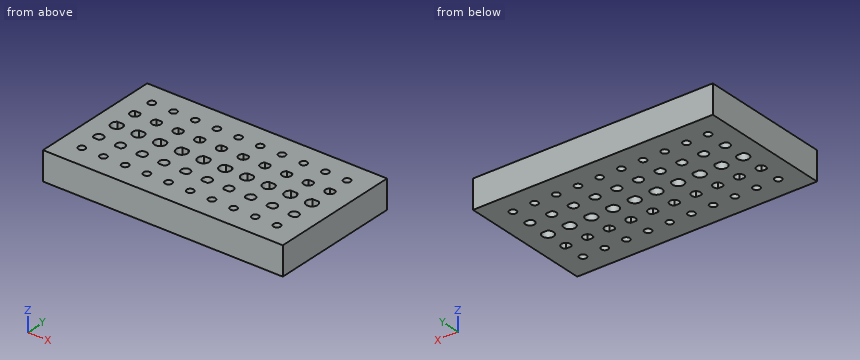
from build123d import *

# Parameters (mm, degrees)
F1_W     = 210
F1_H     = 116
F1_R     = 3.05
F2_DEPTH = 25


with BuildPart() as f2:
    # F1 (on face) → F2 (new body)
    with BuildSketch(Plane.XY):
        with Locations((105, 58)):
            Rectangle(F1_W, F1_H)
        with Locations((19, 19)):
            Circle(F1_R, mode=Mode.SUBTRACT)
        with Locations((38, 19)):
            Circle(F1_R, mode=Mode.SUBTRACT)
        with Locations((57, 19)):
            Circle(F1_R, mode=Mode.SUBTRACT)
        with Locations((76, 19)):
            Circle(F1_R, mode=Mode.SUBTRACT)
        with Locations((95, 19)):
            Circle(F1_R, mode=Mode.SUBTRACT)
        with BuildLine():
            Line((21.362954, 34.834728), (16.637046, 34.834728))
            ThreePointArc((16.637046, 34.834728), (19, 41.95), (21.362954, 34.834728))
        make_face(mode=Mode.SUBTRACT)
        with BuildLine():
            Line((40.362954, 34.834728), (35.637046, 34.834728))
            ThreePointArc((35.637046, 34.834728), (38, 41.95), (40.362954, 34.834728))
        make_face(mode=Mode.SUBTRACT)
        with BuildLine():
            ThreePointArc((21.698148, 62.15), (19, 53.05), (16.301852, 62.15))
            Line((16.301852, 62.15), (21.698148, 62.15))
        make_face(mode=Mode.SUBTRACT)
        with BuildLine():
            ThreePointArc((40.698148, 62.15), (38, 53.05), (35.301852, 62.15))
            Line((35.301852, 62.15), (40.698148, 62.15))
        make_face(mode=Mode.SUBTRACT)
        with BuildLine():
            Line((59.362954, 34.834728), (54.637046, 34.834728))
            ThreePointArc((54.637046, 34.834728), (57, 41.95), (59.362954, 34.834728))
        make_face(mode=Mode.SUBTRACT)
        with BuildLine():
            Line((78.362954, 34.834728), (73.637046, 34.834728))
            ThreePointArc((73.637046, 34.834728), (76, 41.95), (78.362954, 34.834728))
        make_face(mode=Mode.SUBTRACT)
        with BuildLine():
            Line((97.362954, 34.834728), (92.637046, 34.834728))
            ThreePointArc((92.637046, 34.834728), (95, 41.95), (97.362954, 34.834728))
        make_face(mode=Mode.SUBTRACT)
        with BuildLine():
            ThreePointArc((59.698148, 62.15), (57, 53.05), (54.301852, 62.15))
            Line((54.301852, 62.15), (59.698148, 62.15))
        make_face(mode=Mode.SUBTRACT)
        with BuildLine():
            ThreePointArc((78.698148, 62.15), (76, 53.05), (73.301852, 62.15))
            Line((73.301852, 62.15), (78.698148, 62.15))
        make_face(mode=Mode.SUBTRACT)
        with BuildLine():
            ThreePointArc((97.698148, 62.15), (95, 53.05), (92.301852, 62.15))
            Line((92.301852, 62.15), (97.698148, 62.15))
        make_face(mode=Mode.SUBTRACT)
        with Locations((114, 19)):
            Circle(F1_R, mode=Mode.SUBTRACT)
        with Locations((133, 19)):
            Circle(F1_R, mode=Mode.SUBTRACT)
        with Locations((152, 19)):
            Circle(F1_R, mode=Mode.SUBTRACT)
        with Locations((171, 19)):
            Circle(F1_R, mode=Mode.SUBTRACT)
        with Locations((190, 19)):
            Circle(F1_R, mode=Mode.SUBTRACT)
        with BuildLine():
            Line((116.362954, 34.834728), (111.637046, 34.834728))
            ThreePointArc((111.637046, 34.834728), (114, 41.95), (116.362954, 34.834728))
        make_face(mode=Mode.SUBTRACT)
        with BuildLine():
            Line((135.362954, 34.834728), (130.637046, 34.834728))
            ThreePointArc((130.637046, 34.834728), (133, 41.95), (135.362954, 34.834728))
        make_face(mode=Mode.SUBTRACT)
        with BuildLine():
            Line((154.362954, 34.834728), (149.637046, 34.834728))
            ThreePointArc((149.637046, 34.834728), (152, 41.95), (154.362954, 34.834728))
        make_face(mode=Mode.SUBTRACT)
        with BuildLine():
            ThreePointArc((116.698148, 62.15), (114, 53.05), (111.301852, 62.15))
            Line((111.301852, 62.15), (116.698148, 62.15))
        make_face(mode=Mode.SUBTRACT)
        with BuildLine():
            ThreePointArc((135.698148, 62.15), (133, 53.05), (130.301852, 62.15))
            Line((130.301852, 62.15), (135.698148, 62.15))
        make_face(mode=Mode.SUBTRACT)
        with BuildLine():
            ThreePointArc((154.698148, 62.15), (152, 53.05), (149.301852, 62.15))
            Line((149.301852, 62.15), (154.698148, 62.15))
        make_face(mode=Mode.SUBTRACT)
        with BuildLine():
            Line((173.362954, 34.834728), (168.637046, 34.834728))
            ThreePointArc((168.637046, 34.834728), (171, 41.95), (173.362954, 34.834728))
        make_face(mode=Mode.SUBTRACT)
        with BuildLine():
            Line((192.362954, 34.834728), (187.637046, 34.834728))
            ThreePointArc((187.637046, 34.834728), (190, 41.95), (192.362954, 34.834728))
        make_face(mode=Mode.SUBTRACT)
        with BuildLine():
            ThreePointArc((173.698148, 62.15), (171, 53.05), (168.301852, 62.15))
            Line((168.301852, 62.15), (173.698148, 62.15))
        make_face(mode=Mode.SUBTRACT)
        with BuildLine():
            ThreePointArc((192.698148, 62.15), (190, 53.05), (187.301852, 62.15))
            Line((187.301852, 62.15), (192.698148, 62.15))
        make_face(mode=Mode.SUBTRACT)
        with BuildLine():
            ThreePointArc((21.362954, 81.165272), (19, 74.05), (16.637046, 81.165272))
            Line((16.637046, 81.165272), (21.362954, 81.165272))
        make_face(mode=Mode.SUBTRACT)
        with BuildLine():
            ThreePointArc((40.362954, 81.165272), (38, 74.05), (35.637046, 81.165272))
            Line((35.637046, 81.165272), (40.362954, 81.165272))
        make_face(mode=Mode.SUBTRACT)
        with BuildLine():
            ThreePointArc((59.362954, 81.165272), (57, 74.05), (54.637046, 81.165272))
            Line((54.637046, 81.165272), (59.362954, 81.165272))
        make_face(mode=Mode.SUBTRACT)
        with BuildLine():
            ThreePointArc((78.362954, 81.165272), (76, 74.05), (73.637046, 81.165272))
            Line((73.637046, 81.165272), (78.362954, 81.165272))
        make_face(mode=Mode.SUBTRACT)
        with BuildLine():
            ThreePointArc((97.362954, 81.165272), (95, 74.05), (92.637046, 81.165272))
            Line((92.637046, 81.165272), (97.362954, 81.165272))
        make_face(mode=Mode.SUBTRACT)
        with Locations((19, 97)):
            Circle(F1_R, mode=Mode.SUBTRACT)
        with Locations((38, 97)):
            Circle(F1_R, mode=Mode.SUBTRACT)
        with Locations((57, 97)):
            Circle(F1_R, mode=Mode.SUBTRACT)
        with Locations((76, 97)):
            Circle(F1_R, mode=Mode.SUBTRACT)
        with Locations((95, 97)):
            Circle(F1_R, mode=Mode.SUBTRACT)
        with BuildLine():
            ThreePointArc((116.362954, 81.165272), (114, 74.05), (111.637046, 81.165272))
            Line((111.637046, 81.165272), (116.362954, 81.165272))
        make_face(mode=Mode.SUBTRACT)
        with BuildLine():
            ThreePointArc((135.362954, 81.165272), (133, 74.05), (130.637046, 81.165272))
            Line((130.637046, 81.165272), (135.362954, 81.165272))
        make_face(mode=Mode.SUBTRACT)
        with BuildLine():
            ThreePointArc((154.362954, 81.165272), (152, 74.05), (149.637046, 81.165272))
            Line((149.637046, 81.165272), (154.362954, 81.165272))
        make_face(mode=Mode.SUBTRACT)
        with BuildLine():
            ThreePointArc((173.362954, 81.165272), (171, 74.05), (168.637046, 81.165272))
            Line((168.637046, 81.165272), (173.362954, 81.165272))
        make_face(mode=Mode.SUBTRACT)
        with BuildLine():
            ThreePointArc((192.362954, 81.165272), (190, 74.05), (187.637046, 81.165272))
            Line((187.637046, 81.165272), (192.362954, 81.165272))
        make_face(mode=Mode.SUBTRACT)
        with Locations((114, 97)):
            Circle(F1_R, mode=Mode.SUBTRACT)
        with Locations((133, 97)):
            Circle(F1_R, mode=Mode.SUBTRACT)
        with Locations((152, 97)):
            Circle(F1_R, mode=Mode.SUBTRACT)
        with Locations((171, 97)):
            Circle(F1_R, mode=Mode.SUBTRACT)
        with Locations((190, 97)):
            Circle(F1_R, mode=Mode.SUBTRACT)
    extrude(amount=F2_DEPTH)


solid = f2.part
Could you check a few things on this model? Use its own coordinates, in mm. Round coordinates to 2 decimals unless told otherwise and drop trailing zeros. Order: outer loops, then holes, each group sorted by start corner. A loop starts at its lowest first (then second) coordinate and runs counter-clockwise, first axis right, second up.
Q1. Imagine slicing it at B-B, the plane y = 19. State how many separate pieces and enclosed holes the cut face has, then the cut area to 4 significant figures.
Geometry says:
separate pieces: 11
enclosed holes: 0
area: 3,725 mm2
Q2. Please list where these lines run through material, in increasing order: probe 1 along Y at (x, z) = (95, 9); probe 2 along Y at (x, z) = (131, 9.5).
Geometry says:
probe 1: y = 0 to 15.95, 22.05 to 34.83, 41.95 to 53.05, 62.15 to 74.05, 81.17 to 93.95, 100.05 to 116
probe 2: y = 0 to 16.7, 21.3 to 34.83, 41.41 to 53.47, 62.15 to 74.59, 81.17 to 94.7, 99.3 to 116
Q3. Imagine slicing it at A-A, the plane x = 133. List the corners of the cut face in (y, z) for me, then the cut area to 3 significant figures.
Geometry says:
outline: (0, 0) - (15.95, 0) - (15.95, 25) - (0, 25) - close; (22.05, 0) - (34.83, 0) - (34.83, 25) - (22.05, 25) - close; (41.95, 0) - (53.05, 0) - (53.05, 25) - (41.95, 25) - close; (62.15, 0) - (74.05, 0) - (74.05, 25) - (62.15, 25) - close; (81.17, 0) - (93.95, 0) - (93.95, 25) - (81.17, 25) - close; (100.05, 0) - (116, 0) - (116, 25) - (100.05, 25) - close
area: 2,010 mm2
